from build123d import *

# Parameters (mm, degrees)
SKETCH1_R           = 15
BOSS_EXTRUDE1_DEPTH = 30
SKETCH2_R           = 1.5
BOSS_EXTRUDE2_DEPTH = 10
SKETCH3_W           = 2
SKETCH3_H           = 4
BOSS_EXTRUDE3_DEPTH = 5


with BuildPart() as part:
    # Sketch1 → Boss-Extrude1 (new body)
    with BuildSketch(Plane.XY):
        Circle(SKETCH1_R)
    extrude(amount=BOSS_EXTRUDE1_DEPTH)

    # Sketch2 → Boss-Extrude2 (add)
    with BuildSketch(Plane.XY.offset(30)):
        Circle(SKETCH2_R)
    extrude(amount=BOSS_EXTRUDE2_DEPTH)

    # Sketch3 → Boss-Extrude3 (add)
    with BuildSketch(Plane(origin=(0, 0, 0), x_dir=(-1, 0, 0), z_dir=(0, 0, -1))):
        with Locations((-6, 0.376613429)):
            Rectangle(SKETCH3_W, SKETCH3_H)
        with Locations((6, 0.376613429)):
            Rectangle(SKETCH3_W, SKETCH3_H)
    extrude(amount=BOSS_EXTRUDE3_DEPTH)


solid = part.part
Input: part model. Units: mm. Frame: model coordinates. A direction names the side the tool comes from. Give positions to 0.01 mm unless a question says otherwise; leave off trailing zeros. Loops run counter-clockwise (first coordinate to the right, second up) from the corner with the lowest first, then second, coordinate; pieces in that order, holes last. Notation, with made-up numbers: (30.5, 82.25) - (45.5, 82.25) arc R20 ccw to (45.5, 120.25) - close; hole circle Ø6 at (60, 57.25). An arc over 180 degrees is marked (long way). Use CSV: the item, a comma, the result in double quotes. Start each with the question number.
Item 1: Section C-C on z = 37. Return loops of the section in (x, y), then the cut area to 3 significant figures.
Item 2: Section A-A on x = 0. Return loops of the section in (y, z).
Item 3: Section D-D on z = 3. Return loops of the section in (x, y).
Item 4: Mould query, pull axis X, two halves, no side actions, for faces 4 (the flat face through (0, 0, 40)), 5 (the flat face through (5, 0, -2)), 6 (the flat face through (-5, 0, -2)), 7 (the flat face through (7, 0, -2)). Classes: pulls with the +X half, pulls with the -X half, needs draft (parallel to the pull), parting line crosses it, or undercut.
Item 5: Line query: line 1 (Z direction, x = -11, y = -8.5); line 2 (X direction, y = -4, z = 11); line 3 (Y direction, x = 1.5, z = 20.5). Output: solid intervals per line, ascending.
Item 6: Reachability of faces 1 (the flat face through (-7, 0, -2)), 2 (the flat face through (-6, 2.377, -2)), 3 (the flat face through (6, -1.623, -2)) from +Z, -Z, +X, -X, +Y, -Y: full face, straight path, thin tool, end or side. Return the list, or none.
Item 7: Section B-B on y = 0. Return loops of the section in (x, z), then the cut area to 3 significant figures.
Item 8: Contact query for flat-ended pins moving along their axis: P1, Ø0.6, axis at x = -6, z = -2.5, coming from the -Y side; P2, Ø2, axis at y = 1.5, z = -3.5, coming from the -X side; P3, Ø6, axis at x = 8.5, y = -3, coming from the -Z side; P4, Ø4, axis at x = 2.5, z = 3, coming from the +Y side. Output: stop coordinate, or through.
Ans:
1,outline,"circle Ø3 at (0, 0)"
1,area,"7.07 mm2"
2,outline,"(-15, 0) - (15, 0) - (15, 30) - (1.5, 30) - (1.5, 40) - (-1.5, 40) - (-1.5, 30) - (-15, 30) - close"
3,outline,"circle Ø30 at (0, 0)"
4,face 4,"needs draft"
4,face 5,"undercut"
4,face 6,"undercut"
4,face 7,"pulls with the +X half"
5,line 1,"z = 0 to 30"
5,line 2,"x = -14.46 to 14.46"
5,line 3,"y = -14.92 to 14.92"
6,face 1,"-Z, -X, +Y, -Y"
6,face 2,"-Z, +X, -X, +Y"
6,face 3,"-Z, +X, -X, -Y"
7,outline,"(-15, 0) - (-7, 0) - (-7, -5) - (-5, -5) - (-5, 0) - (5, 0) - (5, -5) - (7, -5) - (7, 0) - (15, 0) - (15, 30) - (1.5, 30) - (1.5, 40) - (-1.5, 40) - (-1.5, 30) - (-15, 30) - close"
7,area,"950 mm2"
8,P1,"stops at y = -1.62"
8,P2,"stops at x = -7"
8,P3,"stops at z = -5"
8,P4,"stops at y = 14.99"
